CAD build for the part. Positions are in the model's coordinates, mm. Coordinates: 2 decimals unless noted, no trailing zeros. Write each loop counter-clockwise with the first axis right and the second up, starting at its lowest first coordinate (ties: lowest second). Pieces come first, ordered by that corner, then holes. Notation, with made-up numbers: (62.5, -37.5) -> (121.5, -37.5) arc R20 ccw to (121.5, -21.5) -> close; hole circle Ø6 at (73.25, -27.75). An arc over 180 degrees is marked (long way). Answer as CSV lines item,"result".
```python
from build123d import *

# Parameters (mm, degrees)
F1_DEPTH = 6.35
F3_DEPTH = 19.05
F4_DEPTH = 6.351


with BuildPart() as f1:
    # F0 (on Top) → F1 (new body)
    with BuildSketch(Plane.XY):
        Polygon((-19.05, 0), (0, 0), (0, 25.4), (-31.75, 25.4), (-31.75, 12.7), align=None)
    extrude(amount=F1_DEPTH)

    # F2 (on face) → F3 (join)
    with BuildSketch(Plane.XY.offset(6.35)):
        with BuildLine():
            ThreePointArc((0, 0), (8.9802561211, 3.7197438789), (12.7, 12.7))
            ThreePointArc((12.7, 12.7), (8.9802561211, 21.6802561211), (0, 25.4))
            Line((0, 25.4), (0, 19.05))
            ThreePointArc((0, 19.05), (4.4901280605, 17.1901280605), (6.35, 12.7))
            ThreePointArc((6.35, 12.7), (4.4901280605, 8.2098719395), (0, 6.35))
            Line((0, 6.35), (0, 0))
        make_face()
        with BuildLine():
            Line((0, 19.05), (0, 25.4))
            ThreePointArc((0, 25.4), (-12.7, 12.7), (0, 0))
            Line((0, 0), (0, 6.35))
            ThreePointArc((0, 6.35), (-6.35, 12.7), (0, 19.05))
        make_face()
    extrude(amount=-F3_DEPTH)

    # F4 (cut, through all): a face of the model
    f4_faces = [f1.faces().sort_by_distance(p)[0] for p in [
        (-2.695023703, 12.7, 0),
    ]]
    extrude(f4_faces, amount=-F4_DEPTH, mode=Mode.SUBTRACT)


solid = f1.part
```
Item 1: Two-plate mould, pull along X, no slides. Class faces 1 (the cylindrical face through (-0.279, 6.356, -3.308)), 2 (the flat face through (-31.75, 19, 3)), 3 (the flat face through (-16, 25.4, 3)): pulls with the +X half, pulls with the -X half, needs draft (parallel to the pull), parting line crosses it, or undercut.
Answer below:
face 1,"undercut"
face 2,"pulls with the -X half"
face 3,"needs draft"
Item 2: Wall check: line 1 (X direction, y = 12.7, z = -2); line 2 (X direction, y = 12.7, z = 0.25); line 3 (Z direction, x = -14, y = 1.25). Give the ranges that are in metal, low to high. Write a range as from..to.
Answer below:
line 1,"x = -12.7..-6.35, 6.35..12.7"
line 2,"x = -31.75..-6.35, 6.35..12.7"
line 3,"z = 0..6.35"
Item 3: Saw through at D-D on y = 21.25. Give the cut face in (x, z), and give its area (3 significant figures).
Answer below:
outline,"(-31.75, 0) -> (-9.39, 0) -> (-9.39, -12.7) -> (9.39, -12.7) -> (9.39, 6.35) -> (-31.75, 6.35) -> close"
area,"500 mm2"
Item 4: Saw through at B-B on x = 0.5. Give the cut face in (y, z), and give its area (3 significant figures).
Answer below:
outline,"(0.01, -12.7) -> (6.37, -12.7) -> (6.37, 6.35) -> (0.01, 6.35) -> close; (19.03, -12.7) -> (25.39, -12.7) -> (25.39, 6.35) -> (19.03, 6.35) -> close"
area,"242 mm2"
Item 5: Saw through at A-A on z = 4. Give the cut face in (x, y), and give its area (3 significant figures).
Answer below:
outline,"(-31.75, 12.7) -> (-19.05, 0) -> (0, 0) arc R12.7 ccw to (0, 25.4) -> (-31.75, 25.4) -> close; hole circle Ø12.7 at (0, 12.7)"
area,"852 mm2"
Item 6: Saw through at C-C on y = 18.5. Give the cut face in (x, z), and give its area (3 significant figures).
Answer below:
outline,"(-31.75, 0) -> (-11.3, 0) -> (-11.3, -12.7) -> (-2.59, -12.7) -> (-2.59, 6.35) -> (-31.75, 6.35) -> close; (2.59, -12.7) -> (11.3, -12.7) -> (11.3, 6.35) -> (2.59, 6.35) -> close"
area,"462 mm2"
